The listing builds one solid part. Answer for the finished solid, in the listing's coordinates (mm). Round coordinates to 2 decimals unless told otherwise and drop trailing zeros. Write each loop counter-clockwise with the first axis right and the second up, starting at its lowest first coordinate (ties: lowest second). Pieces come first, ordered by that corner, then holes.
(1) Find the intervals of material crossed by probe 1 along Y at (x, z) = (0, -15.95); probe 2 along X at (y, z) = (0, 15.85); probe 3 along Z at (x, y) = (-0.1, -1.3), in increasing order.
(2) Each of these flat-tipped pins is pushed along its axis until it touches: pin 1 Ø0.8 at (x, y) = (0.5, 0.5) entering from +Z; pin 2 Ø2 at (x, y) = (-2, 1.5) entering from +Z; pin 3 Ø1.2 at (x, y) = (0, -0.5) entering from -Z. Where does it stop, or does it pass through?
(3) A cutting plane is placed at B-B, the plane x = 0. Give the vertices of the cut face in (y, z), and give its area (3 significant figures).
(4) A cutting plane is placed at A-A, the plane z = -8.5. Give the vertices of the cut face in (x, y) (3 decimals).
from build123d import *

# Parameters (mm, degrees)
SKETCH4_R           = 1.75
BOSS_EXTRUDE1_DEPTH = 18.5
SKETCH5_OUTSIDE_W   = 146.91
SKETCH5_OUTSIDE_H   = 146.214
SKETCH5_OUTSIDE_R   = 2.1375
CUT_EXTRUDE1_DEPTH  = 38.159285515
CUT_EXTRUDE1_DRAFT  = -60
SKETCH6_OUTSIDE_W   = 146.91
SKETCH6_OUTSIDE_H   = 146.214
SKETCH6_OUTSIDE_R   = 2.1375
CUT_EXTRUDE2_DEPTH  = 38.159285515
CUT_EXTRUDE2_DRAFT  = -60
FILLET1_R           = 0.45


with BuildPart() as part:
    # Sketch3 → Revolve1 (revolve)
    with BuildSketch(Plane(origin=(0, 0, 0), x_dir=(0, 0, -1), z_dir=(1, 0, 0))):
        Polygon((-18.243800818, 1.25), (-13.7, 1.25), (-13.7, 0), (13.7, 0), (13.7, 1.25), (18.243800818, 1.25), (18.5, 1.69375), (18.5, 2.25), (0, 2.25), (-18.5, 2.25), (-18.5, 1.69375), align=None)
        Polygon((-18.243800818, 1.25), (-13.7, 1.25), (-13.7, 0), (13.7, 0), (13.7, 1.25), (18.243800818, 1.25), (18.5, 1.69375), (18.5, 2.25), (0, 2.25), (-18.5, 2.25), (-18.5, 1.69375), align=None)
    revolve(axis=Axis((0, 0, 13.7), (0, 0, 1)))

    # Sketch4 → Boss-Extrude1 (add, symmetric)
    with BuildSketch(Plane.XY):
        Polygon((-1.299038106, 2.25), (-2.598076211, 0), (-1.299038106, -2.25), (1.299038106, -2.25), (2.598076211, 0), (1.299038106, 2.25), align=None)
        Circle(SKETCH4_R, mode=Mode.SUBTRACT)
    extrude(amount=BOSS_EXTRUDE1_DEPTH, both=True)


with BuildPart() as cut_extrude1_tool:
    # Sketch5 outside → Cut-Extrude1 (with draft: the straight prism first)
    with BuildSketch(Plane.XY.offset(18.5)):
        Rectangle(SKETCH5_OUTSIDE_W, SKETCH5_OUTSIDE_H)
        Circle(SKETCH5_OUTSIDE_R, mode=Mode.SUBTRACT)
    extrude(amount=-CUT_EXTRUDE1_DEPTH)
    # Cut-Extrude1: the draft: its side faces are tilted about the plane it starts from
    cut_extrude1_sides = [cut_extrude1_tool.faces().sort_by_distance(p)[0] for p in [
        (0, -73.107, -0.579642758),
        (73.455, 0, -0.579642758),
        (0, 73.107, -0.579642758),
        (-73.455, 0, -0.579642758),
        (-2.1375, 0, -0.579642758),
    ]]
    draft(cut_extrude1_sides, Plane.XY.offset(18.5), CUT_EXTRUDE1_DRAFT)


with BuildPart() as part_1:
    add(part.part)

    # Cut-Extrude1: cut by cut_extrude1_tool
    add(cut_extrude1_tool.part, mode=Mode.SUBTRACT)


with BuildPart() as cut_extrude2_tool:
    # Sketch6 outside → Cut-Extrude2 (with draft: the straight prism first)
    with BuildSketch(Plane(origin=(0, 0, -18.5), x_dir=(-1, 0, 0), z_dir=(0, 0, -1))):
        Rectangle(SKETCH6_OUTSIDE_W, SKETCH6_OUTSIDE_H)
        Circle(SKETCH6_OUTSIDE_R, mode=Mode.SUBTRACT)
    extrude(amount=-CUT_EXTRUDE2_DEPTH)
    # Cut-Extrude2: the draft: its side faces are tilted about the plane it starts from
    cut_extrude2_sides = [cut_extrude2_tool.faces().sort_by_distance(p)[0] for p in [
        (0, -73.107, 0.579642758),
        (-73.455, 0, 0.579642758),
        (0, 73.107, 0.579642758),
        (73.455, 0, 0.579642758),
        (2.1375, 0, 0.579642758),
    ]]
    draft(cut_extrude2_sides, Plane(origin=(0, 0, -18.5), x_dir=(-1, 0, 0), z_dir=(0, 0, -1)), CUT_EXTRUDE2_DRAFT)


with BuildPart() as part_2:
    add(part_1.part)

    # Cut-Extrude2: cut by cut_extrude2_tool
    add(cut_extrude2_tool.part, mode=Mode.SUBTRACT)

    # Fillet1
    # the kernel refuses this fillet: 0.45 mm, written as the material it takes off along each edge
    with BuildSketch(Plane(origin=(1.299038106, 2.25, 18.883605253), x_dir=(-1, 0, 0), z_dir=(0, 0, -1)), Plane(origin=(-1.299038106, 2.25, 18.883605253), x_dir=(-0.49999999999999967, -0.8660254037844387, 0), z_dir=(0, 0, -1))) as fillet1_piece_1:
        with BuildLine():
            CenterArc((FILLET1_R * 0.57735026919, -FILLET1_R), FILLET1_R, 90, 60)
            Line((-FILLET1_R * 0.288675134595, -FILLET1_R * 0.5), (0, 0))
            Line((0, 0), (FILLET1_R * 0.57735026919, 0))
        make_face()
    extrude(amount=37.767210506, mode=Mode.SUBTRACT)
    with BuildSketch(Plane(origin=(-2.598076211, 0, -18.883605253), x_dir=(0.5000000000000006, -0.8660254037844384, 0), z_dir=(0, 0, 1)), Plane(origin=(-1.299038106, -2.25, -18.883605253), x_dir=(1, 0, 0), z_dir=(0, 0, 1)), Plane(origin=(1.299038106, -2.25, -18.883605253), x_dir=(0.49999999999999967, 0.8660254037844387, 0), z_dir=(0, 0, 1)), Plane(origin=(2.598076211, 0, 18.883605253), x_dir=(-0.5, -0.8660254037844388, 0), z_dir=(0, 0, -1))) as fillet1_piece_2:
        with BuildLine():
            CenterArc((FILLET1_R * 0.57735026919, FILLET1_R), FILLET1_R, 210, 60)
            Line((-FILLET1_R * 0.288675134595, FILLET1_R * 0.5), (0, 0))
            Line((0, 0), (FILLET1_R * 0.57735026919, 0))
        make_face()
    extrude(amount=37.767210506, mode=Mode.SUBTRACT)


solid = part_2.part
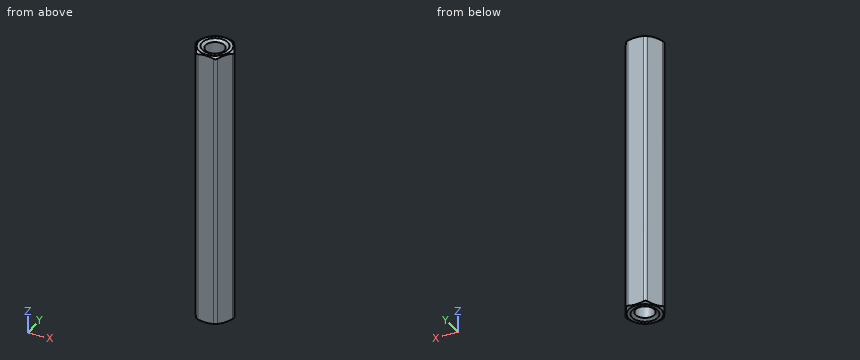
Solutions:
1. probe 1: y = -2.25 to -1.25, 1.25 to 2.25
1. probe 2: x = -2.53 to -1.25, 1.25 to 2.53
1. probe 3: z = -18.27 to 18.27
2. pin 1: stops at z = 13.7
2. pin 2: stops at z = 18.5
2. pin 3: stops at z = -13.7
3. outline: (-2.25, -18.44) - (-2.14, -18.5) - (-1.69, -18.5) - (-1.25, -18.24) - (-1.25, -13.7) - (1.25, -13.7) - (1.25, -18.24) - (1.69, -18.5) - (2.14, -18.5) - (2.25, -18.44) - (2.25, 18.44) - (2.14, 18.5) - (1.69, 18.5) - (1.25, 18.24) - (1.25, 13.7) - (-1.25, 13.7) - (-1.25, 18.24) - (-1.69, 18.5) - (-2.14, 18.5) - (-2.25, 18.44) - close
3. area: 142 mm2
4. outline: (-2.468, -0.225) - (-1.429, -2.025) arc R0.45 ccw to (-1.039, -2.25) - (1.039, -2.25) arc R0.45 ccw to (1.429, -2.025) - (2.468, -0.225) arc R0.45 ccw to (2.468, 0.225) - (1.429, 2.025) arc R0.45 ccw to (1.039, 2.25) - (-1.039, 2.25) arc R0.45 ccw to (-1.429, 2.025) - (-2.468, 0.225) arc R0.45 ccw to start
